Geometry check sheet. Reference: the model listing, model coordinates, mm. A direction names the side the tool comes from. Give positions to 0.01 mm unless a question says otherwise; leave off trailing zeros. Loops run counter-clockwise (first coordinate to the right, second up) from the corner with the lowest first, then second, coordinate; pieces in that order, holes last.
1. Go/stop test with flat-tipped pins: pin 1 Ø6 at (x, y) = (76.5, -45.5) entering from -Z; pin 2 Ø1 at (y, z) = (-107.5, 417.5) entering from +X; pin 3 Ø2 at (y, z) = (56.5, 871) entering from -X. Record where each tip stops, or that it passes through.
2. Cross-section at A-A, the plane x = 177.8. Record the cut outline in (y, z).
3. Tool access check on faces 4 (the flat face through (209.55, 108, 521)), 5 (the cylindrical face through (-166.068, 103.086, 38.633)), 6 (the flat face through (-146.05, -2, 520)), 7 (the flat face through (44.45, -98, 31)), 8 (the flat face through (-77, -57.15, 31)). Record the directions out of +Z, -Z, +X, -X, +Y, -Y that give a thin tool (end or side, any length) a straight path to the whole face; none if there is none.
4. Cross-section at C-C, the plane x = 76.2. Record the cut outline in (y, z).
5. Material ranges on L1, parallel to X at y = 127.5, z = 670.5; L2, parallel to Y at x = 0, z = 1043.5; L3, parallel to X at y = -56, z = 256, recorded low to high.
6. Cross-section at B-B, the plane y = -95.25. Record the cut outline in (x, z), plus the area to 3 significant figures.
7. Cross-section at D-D, the plane z = 821.5. Record the cut outline in (x, y), plus the area to 3 significant figures.
8. Release check for a two-part mould opening along Y. For faces 1 (the cylindrical face through (-2.75, 82.85, 31.31)), 2 (the flat face through (-247.65, 108, 520)), 3 (the flat face through (-220, 76.2, 520)) record: +Y half, -Y half, draft (parallel to the pull), parting line (faces both ways), or undercut.
from build123d import *

# Parameters (mm, degrees)
SKETCH1_R           = 12.7
BOSS_EXTRUDE1_DEPTH = 63.5
BOSS_EXTRUDE2_REACH = 323.601
SKETCH2_W           = 38.1
SKETCH2_H           = 939.8
SKETCH3_W           = 38.1
SKETCH3_H           = 279.4
SKETCH3_W_2         = 215.9
SKETCH3_R           = 12.7
BOSS_EXTRUDE3_DEPTH = 50.8
CUT_EXTRUDE1_REACH  = 1075.3
SKETCH4_R           = 19.05
SKETCH5_W           = 38.1
SKETCH5_H           = 63.5
SKETCH5_W_2         = 63.5
SKETCH5_R           = 12.7
BOSS_EXTRUDE4_DEPTH = 76.2
BOSS_EXTRUDE5_START = -977.9
SKETCH5_3_W         = 38.1
SKETCH5_3_H         = 63.5
SKETCH5_3_W_2       = 63.5
SKETCH5_3_R         = 12.7
BOSS_EXTRUDE5_DEPTH = 76.2
BOSS_EXTRUDE6_START = -977.9
SKETCH5_4_W         = 38.1
SKETCH5_4_H         = 63.5
BOSS_EXTRUDE6_DEPTH = 901.7


with BuildPart() as part:
    # Sketch1 → Boss-Extrude1 (new body)
    with BuildSketch(Plane.XY):
        Polygon((146.05, 139.7), (-146.05, 139.7), (-146.05, -139.7), (-44.45, -139.7), (-44.45, -57.15), (-111.125, -57.15), (-111.125, 57.15), (111.125, 57.15), (111.125, -57.15), (44.45, -57.15), (44.45, -139.7), (146.05, -139.7), align=None)
        with Locations((-76.2, -95.25)):
            Circle(SKETCH1_R, mode=Mode.SUBTRACT)
        with Locations((76.2, -95.25)):
            Circle(SKETCH1_R, mode=Mode.SUBTRACT)
        with Locations((0, 95.25)):
            Circle(SKETCH1_R, mode=Mode.SUBTRACT)
    extrude(amount=BOSS_EXTRUDE1_DEPTH)

    # Boss-Extrude2: up to this face of the body (flat: up to its plane)
    boss_extrude2_end = Plane(part.part.faces().sort_by_distance((-95.25, -139.7, 31.75))[0])
    # Sketch2 → Boss-Extrude2 (add, up to the picked face)
    with BuildSketch(Plane(origin=(0, 139.7, 0), x_dir=(1, 0, 0), z_dir=(0, 1, 0)), mode=Mode.PRIVATE) as boss_extrude2_sk1:
        with Locations((-127, -533.4)):
            Rectangle(SKETCH2_W, SKETCH2_H)
    boss_extrude2_tool1 = split(extrude(boss_extrude2_sk1.sketch, amount=-BOSS_EXTRUDE2_REACH, mode=Mode.PRIVATE), bisect_by=boss_extrude2_end, keep=Keep.BOTH, mode=Mode.PRIVATE)
    # Sketch2 → Boss-Extrude2 (add, up to the picked face)
    with BuildSketch(Plane(origin=(0, 139.7, 0), x_dir=(1, 0, 0), z_dir=(0, 1, 0)), mode=Mode.PRIVATE) as boss_extrude2_sk2:
        with Locations((127, -533.4)):
            Rectangle(SKETCH2_W, SKETCH2_H)
    boss_extrude2_tool2 = split(extrude(boss_extrude2_sk2.sketch, amount=-BOSS_EXTRUDE2_REACH, mode=Mode.PRIVATE), bisect_by=boss_extrude2_end, keep=Keep.BOTH, mode=Mode.PRIVATE)
    add(boss_extrude2_tool1.solids().sort_by(Axis((-127, 139.7, 533.4), (0, -1, 0)))[0])
    add(boss_extrude2_tool2.solids().sort_by(Axis((127, 139.7, 533.4), (0, -1, 0)))[0])

    # Sketch3 → Boss-Extrude3 (add)
    # profile 1 of 3: a face of its own
    with BuildSketch(Plane.XY.offset(1003.3)):
        with Locations((-127, 0)):
            Rectangle(SKETCH3_W, SKETCH3_H)
    # profile 2 of 3: a face of its own
    with BuildSketch(Plane.XY.offset(1003.3)):
        Rectangle(SKETCH3_W_2, SKETCH3_H)
        with Locations((-76.2, -95.25)):
            Circle(SKETCH3_R, mode=Mode.SUBTRACT)
        with Locations((76.2, -95.25)):
            Circle(SKETCH3_R, mode=Mode.SUBTRACT)
        with Locations((0, 95.25)):
            Circle(SKETCH3_R, mode=Mode.SUBTRACT)
    # profile 3 of 3: a face of its own
    with BuildSketch(Plane.XY.offset(1003.3)):
        with Locations((127, 0)):
            Rectangle(SKETCH3_W, SKETCH3_H)
    extrude(amount=BOSS_EXTRUDE3_DEPTH)

    # Sketch4 → Cut-Extrude1 (cut, up to next)
    with BuildSketch(Plane.XY.offset(1054.1), mode=Mode.PRIVATE) as cut_extrude1_sk1:
        Circle(SKETCH4_R)
    cut_extrude1_tool1 = extrude(cut_extrude1_sk1.sketch, amount=-CUT_EXTRUDE1_REACH, mode=Mode.PRIVATE) & part.part
    add(cut_extrude1_tool1.solids().sort_by_distance((0, 0, 1054.1))[0], mode=Mode.SUBTRACT)

    # Sketch5 → Boss-Extrude4 (add)
    # profile 1 of 4: a face of its own
    with BuildSketch(Plane.XY.offset(1054.1)):
        with Locations((228.6, 107.95)):
            Rectangle(SKETCH5_W, SKETCH5_H)
    # profile 2 of 4: a face of its own
    with BuildSketch(Plane.XY.offset(1054.1)):
        with Locations((177.8, 107.95)):
            Rectangle(SKETCH5_W_2, SKETCH5_H)
        with Locations((177.8, 107.95)):
            Circle(SKETCH5_R, mode=Mode.SUBTRACT)
    # profile 3 of 4: a face of its own
    with BuildSketch(Plane.XY.offset(1054.1)):
        with Locations((-228.6, 107.95)):
            Rectangle(SKETCH5_W, SKETCH5_H)
    # profile 4 of 4: a face of its own
    with BuildSketch(Plane.XY.offset(1054.1)):
        with Locations((-177.8, 107.95)):
            Rectangle(SKETCH5_W_2, SKETCH5_H)
        with Locations((-177.8, 107.95)):
            Circle(SKETCH5_R, mode=Mode.SUBTRACT)
    extrude(amount=-BOSS_EXTRUDE4_DEPTH)

    # Sketch5<3> → Boss-Extrude5 (add)
    # profile 1 of 4: a face of its own
    with BuildSketch(Plane.XY.offset(1054.1).offset(BOSS_EXTRUDE5_START)):
        with Locations((228.6, 107.95)):
            Rectangle(SKETCH5_3_W, SKETCH5_3_H)
    # profile 2 of 4: a face of its own
    with BuildSketch(Plane.XY.offset(1054.1).offset(BOSS_EXTRUDE5_START)):
        with Locations((177.8, 107.95)):
            Rectangle(SKETCH5_3_W_2, SKETCH5_3_H)
        with Locations((177.8, 107.95)):
            Circle(SKETCH5_3_R, mode=Mode.SUBTRACT)
    # profile 3 of 4: a face of its own
    with BuildSketch(Plane.XY.offset(1054.1).offset(BOSS_EXTRUDE5_START)):
        with Locations((-228.6, 107.95)):
            Rectangle(SKETCH5_3_W, SKETCH5_3_H)
    # profile 4 of 4: a face of its own
    with BuildSketch(Plane.XY.offset(1054.1).offset(BOSS_EXTRUDE5_START)):
        with Locations((-177.8, 107.95)):
            Rectangle(SKETCH5_3_W_2, SKETCH5_3_H)
        with Locations((-177.8, 107.95)):
            Circle(SKETCH5_3_R, mode=Mode.SUBTRACT)
    extrude(amount=-BOSS_EXTRUDE5_DEPTH)

    # Sketch5<4> → Boss-Extrude6 (add)
    with BuildSketch(Plane.XY.offset(1054.1).offset(BOSS_EXTRUDE6_START)):
        with Locations((-228.6, 107.95)):
            Rectangle(SKETCH5_4_W, SKETCH5_4_H)
        with Locations((228.6, 107.95)):
            Rectangle(SKETCH5_4_W, SKETCH5_4_H)
    extrude(amount=BOSS_EXTRUDE6_DEPTH)


solid = part.part
Result:
1. pin 1: stops at z = 1003.3
1. pin 2: stops at x = 146.05
1. pin 3: stops at x = -146.05
2. outline: (76.2, 0) - (95.25, 0) - (95.25, 76.2) - (76.2, 76.2) - close; (76.2, 977.9) - (95.25, 977.9) - (95.25, 1054.1) - (76.2, 1054.1) - close; (120.65, 0) - (139.7, 0) - (139.7, 76.2) - (120.65, 76.2) - close; (120.65, 977.9) - (139.7, 977.9) - (139.7, 1054.1) - (120.65, 1054.1) - close
3. face 4: +Y, -Y
3. face 5: +Z, -Z
3. face 6: -Y
3. face 7: -Z, -Y
3. face 8: -Z
4. outline: (-139.7, 0) - (-107.95, 0) - (-107.95, 63.5) - (-139.7, 63.5) - close; (-139.7, 1003.3) - (-107.95, 1003.3) - (-107.95, 1054.1) - (-139.7, 1054.1) - close; (-82.55, 0) - (-57.15, 0) - (-57.15, 63.5) - (-82.55, 63.5) - close; (-82.55, 1003.3) - (139.7, 1003.3) - (139.7, 1054.1) - (-82.55, 1054.1) - close; (57.15, 0) - (139.7, 0) - (139.7, 63.5) - (57.15, 63.5) - close
5. L1: x = -247.65 to -209.55, -146.05 to -107.95, 107.95 to 146.05, 209.55 to 247.65
5. L2: y = -139.7 to -19.05, 19.05 to 82.55, 107.95 to 139.7
5. L3: x = -146.05 to -107.95, 107.95 to 146.05
6. outline: (-146.05, 0) - (-88.9, 0) - (-88.9, 63.5) - (-107.95, 63.5) - (-107.95, 1003.3) - (-88.9, 1003.3) - (-88.9, 1054.1) - (-146.05, 1054.1) - close; (-63.5, 0) - (-44.45, 0) - (-44.45, 63.5) - (-63.5, 63.5) - close; (-63.5, 1003.3) - (63.5, 1003.3) - (63.5, 1054.1) - (-63.5, 1054.1) - close; (44.45, 0) - (63.5, 0) - (63.5, 63.5) - (44.45, 63.5) - close; (88.9, 0) - (146.05, 0) - (146.05, 1054.1) - (88.9, 1054.1) - (88.9, 1003.3) - (107.95, 1003.3) - (107.95, 63.5) - (88.9, 63.5) - close
6. area: 93,500 mm2
7. outline: (-247.65, 76.2) - (-209.55, 76.2) - (-209.55, 139.7) - (-247.65, 139.7) - close; (-146.05, -139.7) - (-107.95, -139.7) - (-107.95, 139.7) - (-146.05, 139.7) - close; (107.95, -139.7) - (146.05, -139.7) - (146.05, 139.7) - (107.95, 139.7) - close; (209.55, 76.2) - (247.65, 76.2) - (247.65, 139.7) - (209.55, 139.7) - close
7. area: 26,100 mm2
8. face 1: undercut
8. face 2: draft
8. face 3: -Y half
